```python
from build123d import *

# Parameters (mm, degrees)
SKETCH_1_R           = 7
SKETCH_1_R_2         = 1.5
EXTRUDE_1_DEPTH      = 3
SKETCH_1_3_R         = 7
SKETCH_1_3_R_2       = 4
EXTRUDE_2_DEPTH      = 7
HOLE_WIZARD_M1_6_1_D = 1.25


with BuildPart() as part:
    # Sketch 1 → Extrude 1 (new body)
    with BuildSketch(Plane(origin=(0, 0, 0), x_dir=(1, 0, 0), z_dir=(0, 1, 0))):
        with BuildLine():
            Line((2.4, 7.631513611), (16.05, 3.338787205))
            ThreePointArc((16.05, 3.338787205), (18.5, 0), (16.05, -3.338787205))
            Line((16.05, -3.338787205), (2.4, -7.631513611))
            ThreePointArc((2.4, -7.631513611), (0, -8), (-2.4, -7.631513611))
            Line((-2.4, -7.631513611), (-16.05, -3.338787205))
            ThreePointArc((-16.05, -3.338787205), (-18.5, 0), (-16.05, 3.338787205))
            Line((-16.05, 3.338787205), (-2.4, 7.631513611))
            ThreePointArc((-2.4, 7.631513611), (0, 8), (2.4, 7.631513611))
        make_face()
        with Locations(Location((0, 0, 0), (0, 0, 270))):
            Circle(SKETCH_1_R, mode=Mode.SUBTRACT)
        with Locations(Location((15, 0, 0), (0, 0, 270))):
            Circle(SKETCH_1_R_2, mode=Mode.SUBTRACT)
        with Locations(Location((-15, 0, 0), (0, 0, 270))):
            Circle(SKETCH_1_R_2, mode=Mode.SUBTRACT)
    extrude(amount=EXTRUDE_1_DEPTH)

    # Sketch 1_3 → Extrude 2 (add)
    with BuildSketch(Plane(origin=(0, 0, 0), x_dir=(1, 0, 0), z_dir=(0, 1, 0))):
        with Locations(Location((0, 0, 0), (0, 0, 270))):
            Circle(SKETCH_1_3_R)
        with Locations(Location((0, 0, 0), (0, 0, 270))):
            Circle(SKETCH_1_3_R_2, mode=Mode.SUBTRACT)
    extrude(amount=EXTRUDE_2_DEPTH)

    # Hole Wizard M1.6 _1 (through all)
    with Locations(Plane(origin=(6.99996172, 4.619290958, 0.023149905), x_dir=(-0.003307129319, 0, 0.999994531433), z_dir=(0.999994531433, 0, 0.003307129319))):
        with Locations((0, 0)):
            Hole(HOLE_WIZARD_M1_6_1_D / 2)


solid = part.part
```
Geometry: final body of the model. Coordinates: model frame, mm. A direction names the side the tool comes from. Give positions to 0.01 mm unless a question says otherwise; leave off trailing zeros. Loops run counter-clockwise (first coordinate to the right, second up) from the corner with the lowest first, then second, coordinate; pieces in that order, holes last. Notation, with made-up numbers: (57, 45) -> (70, 45) arc R27 ccw to (70, 69) -> close; hole circle Ø5 at (54.25, 33.5). An arc over 180 degrees is marked (long way). Use one line per item in the form item = value.
Item 1: Section query A-A on y = 2.25. Output: boundary loops of the cut face in (x, z).
A:
outline = (-16.05, -3.34) -> (-2.4, -7.63) arc R8 ccw to (2.4, -7.63) -> (16.05, -3.34) arc R3.5 ccw to (16.05, 3.34) -> (2.4, 7.63) arc R8 ccw to (-2.4, 7.63) -> (-16.05, 3.34) arc R3.5 ccw to start; hole circle Ø3 at (-15, 0); hole circle Ø8 at (0, 0); hole circle Ø3 at (15, 0)
Item 2: Line query: probe 1 along X at (y, z) = (1.5, 0); probe 2 along X at (y, z) = (1.25, -1.25); probe 3 along Y at (x, z) = (-4, 6). Output: solid intervals per line, ascending.
A:
probe_1 = -18.5 to -16.5, -13.5 to -4, 4 to 13.5, 16.5 to 18.5
probe_2 = -18.27 to -15.83, -14.17 to -3.8, 3.8 to 14.17, 15.83 to 18.27
probe_3 = 0 to 3
Item 3: Section query D-D on y = 5.75. Output: boundary loops of the cut face in (x, z), and give its area (3 significant figures).
A:
outline = circle Ø14 at (0, 0); hole circle Ø8 at (0, 0)
area = 104 mm^2
Item 4: Access query for faces 1 (the face through (-9.321, 1.479, -5.455)), 2 (the face through (0, 1, -8)), 3 (the face through (-6.834, 4.972, -1.517)). Directions: +Z, -Z, +X, -X, +Y, -Y. A direction counts if a zero-diameter tool reaches every point of the face in a straight line with its end or side. Return the directions, or none.
A:
face_1 = -Z, -X, +Y, -Y
face_2 = -Z, +Y, -Y
face_3 = +Y
Item 5: Section query C-C on z = 6.5. Output: boundary loops of the cut face in (x, y).
A:
outline = (-6, 0) -> (6, 0) -> (6, 3) -> (2.6, 3) -> (2.6, 7) -> (-2.6, 7) -> (-2.6, 3) -> (-6, 3) -> close
Item 6: Section query B-B on x = -1. Output: boundary loops of the cut face in (y, z), and give its area (3 significant figures).
A:
outline = (0, -7.94) -> (3, -7.94) -> (3, -6.93) -> (7, -6.93) -> (7, -3.87) -> (0, -3.87) -> close; (0, 3.87) -> (7, 3.87) -> (7, 6.93) -> (3, 6.93) -> (3, 7.94) -> (0, 7.94) -> close
area = 48.8 mm^2
Item 7: Draft query along X for faces 4 (the face through (-3.905, 3.451, -0.867)), 5 (the face through (0, 1, 8)), 6 (the face through (-18.5, 1.5, 0.1)), 7 (the face through (16.265, 1.479, 0.806)). Return one class per face: pulls with the +X half, pulls with the -X half, needs draft (parallel to the pull), parting line crosses it, or undercut.
A:
face_4 = undercut
face_5 = parting line crosses it
face_6 = pulls with the -X half
face_7 = undercut
Item 8: Pin query (flat end, axial travel): P1, Ø4, axis at x = -8, y = 1.5, coming from the +Z side; P2, Ø1, axis at y = 2, z = 3, coming from the -X side; P3, Ø1.5, axis at x = -8, z = -5, coming from the +Y side. Return the tip coordinate at first contact, or that it passes through.
A:
P1 = 6.5
P2 = -17.45
P3 = 3
